Read the model definition and answer for the solid it produces. Units are mm, in the model's axes. A direction names the side the tool comes from. Give positions to 0.01 mm unless a question says otherwise; leave off trailing zeros. Loops run counter-clockwise (first coordinate to the right, second up) from the corner with the lowest first, then second, coordinate; pieces in that order, holes last.
(1) Straight lines are drawn through the part: probe 1 along Y at (x, z) = (-13, 12.75); probe 2 along X at (y, z) = (-15, 6); probe 3 along X at (y, z) = (-33.45, 27.5). For each, find the intervals that lie inside material, in ascending order.
(2) Which of the six approach directions +Z, -Z, +X, -X, +Y, -Y give full straight-line access (tool end or side, diameter ignored) to faces 1 (the face through (-14, -33.279, 27)), 2 (the face through (-4.076, -41.895, 27.395)), 3 (the face through (-6.434, 5.9, 3.914))?
(3) Determine the mould class of faces 4 (the face through (0, 25, 10)), 5 (the face through (-1.82, -23.22, 13.41)), 6 (the face through (8, -34.261, 25.7)), 7 (the face through (-15.674, -15.132, 9.86)) for opening direction Y: pulls with the +Y half, pulls with the -Y half, needs draft (parallel to the pull), parting line crosses it, or undercut.
(4) Each of these flat-tipped pins is pushed along its axis until it touches: P1, Ø14, axis at x = -0.5, y = 1.5, coming from the -Z side; P2, Ø6.5, axis at x = 8.5, z = 24.5, coming from the +Y side; P3, Ø3, axis at x = -2, y = -23, coming from the +Z side; P4, Ø13, axis at x = -6, y = 1, coming from the +Z side. Where does it stop, or does it pass through?
(5) Find section C-C, the plane x = -1. Write down the section's boundary in (y, z).
(6) Find section A-A, the plane z = 27.5. State how many separate pieces and enclosed holes the cut face has, then the cut area to 3 significant figures.
(7) Find section B-B, the plane y = -17. Write down the section's boundary in (x, z), then the cut area to 3 significant figures.
(8) Find section D-D, the plane z = 18.5. Write down the section's boundary in (x, y), then the cut area to 3 significant figures.
```python
from build123d import *

# Parameters (mm, degrees)
SKETCH1_W           = 42.62295082
SKETCH1_H           = 50
SKETCH1_R           = 2.677018134
BOSS_EXTRUDE1_DEPTH = 20
SKETCH2_R           = 8.73
CUT_EXTRUDE2_DEPTH  = 7.94
SKETCH3_R           = 2.2
CUT_EXTRUDE3_DEPTH  = 10
CUT_EXTRUDE4_START  = -7
CUT_EXTRUDE4_DEPTH  = 32.460095998
SKETCH7_W           = 42.62295082
SKETCH7_H           = 20
BOSS_EXTRUDE2_DEPTH = 18
SKETCH6_R           = 6.4
CUT_EXTRUDE5_DEPTH  = 52.992105017
BOSS_EXTRUDE5_DEPTH = 15
SKETCH10_R          = 1.55
CUT_EXTRUDE8_DEPTH  = 80.392562524


with BuildPart() as part:
    # Sketch1 → Boss-Extrude1 (new body)
    with BuildSketch(Plane.XY):
        Rectangle(SKETCH1_W, SKETCH1_H)
        with Locations((-13, -15.25)):
            Circle(SKETCH1_R, mode=Mode.SUBTRACT)
        with Locations(Location((13, -15.25, 0), (0, 0, 180))):
            Circle(SKETCH1_R, mode=Mode.SUBTRACT)
        with Locations((13, 15.25)):
            Circle(SKETCH1_R, mode=Mode.SUBTRACT)
        with Locations(Location((-13, 15.25, 0), (0, 0, 180))):
            Circle(SKETCH1_R, mode=Mode.SUBTRACT)
    extrude(amount=BOSS_EXTRUDE1_DEPTH)

    # Sketch2 → Cut-Extrude2 (cut)
    with BuildSketch(Plane.XY):
        Circle(SKETCH2_R)
    extrude(amount=CUT_EXTRUDE2_DEPTH, mode=Mode.SUBTRACT)

    # Sketch3 → Cut-Extrude3 (cut)
    with BuildSketch(Plane(origin=(0, 0, 0), x_dir=(-1, 0, 0), z_dir=(0, 0, -1))):
        with Locations((0, -20)):
            Circle(SKETCH3_R)
    extrude(amount=-CUT_EXTRUDE3_DEPTH, mode=Mode.SUBTRACT)

    # Sketch5 → Cut-Extrude4 (cut, through all)
    with BuildSketch(Plane(origin=(0, 0, 0), x_dir=(-1, 0, 0), z_dir=(0, 0, -1)).offset(CUT_EXTRUDE4_START)):
        Polygon((0, -15.727608008), (-3.7, -17.863804004), (-3.7, -22.136195996), (0, -24.272391992), (3.7, -22.136195996), (3.7, -17.863804004), align=None)
    extrude(amount=-CUT_EXTRUDE4_DEPTH, mode=Mode.SUBTRACT)

    # Sketch7 → Boss-Extrude2 (add)
    with BuildSketch(Plane.XZ.offset(25)):
        with Locations((0, 10)):
            Rectangle(SKETCH7_W, SKETCH7_H)
    extrude(amount=BOSS_EXTRUDE2_DEPTH)

    # Sketch6 → Cut-Extrude5 (cut, through all)
    with BuildSketch(Plane(origin=(0, 0, 0), x_dir=(-1, 0, 0), z_dir=(0, 0, -1))):
        with Locations((3.896856088, -32.824049036)):
            Circle(SKETCH6_R)
    extrude(amount=-CUT_EXTRUDE5_DEPTH, mode=Mode.SUBTRACT)

    # Sketch8 → Boss-Extrude5 (add)
    with BuildSketch(Plane.XY.offset(20)):
        with BuildLine():
            ThreePointArc((-10.280677785, -32.369273769), (-3.896856088, -26.424049036), (2.486965609, -32.369273769))
            Line((2.486965609, -32.369273769), (11.091790538, -32.369273769))
            Line((11.091790538, -32.369273769), (11.091790538, -31.387593744))
            Line((11.091790538, -31.387593744), (5.061469986, -31.387593744))
            ThreePointArc((5.061469986, -31.387593744), (-3.896856088, -23.751287061), (-12.855182162, -31.387593744))
            Line((-12.855182162, -31.387593744), (-18.885502714, -31.387593744))
            Line((-18.885502714, -31.387593744), (-18.885502714, -32.369273769))
            Line((-18.885502714, -32.369273769), (-10.280677785, -32.369273769))
        make_face()
        with BuildLine():
            Line((-10.280677785, -33.278824303), (-18.885502714, -33.278824303))
            Line((-18.885502714, -33.278824303), (-18.885502714, -34.260504328))
            Line((-18.885502714, -34.260504328), (-12.855182162, -34.260504328))
            ThreePointArc((-12.855182162, -34.260504328), (-3.896856088, -41.896811011), (5.061469986, -34.260504328))
            Line((5.061469986, -34.260504328), (11.091790538, -34.260504328))
            Line((11.091790538, -34.260504328), (11.091790538, -33.278824303))
            Line((11.091790538, -33.278824303), (2.486965609, -33.278824303))
            ThreePointArc((2.486965609, -33.278824303), (-3.896856088, -39.224049036), (-10.280677785, -33.278824303))
        make_face()
    extrude(amount=BOSS_EXTRUDE5_DEPTH)

    # Sketch10 → Cut-Extrude8 (cut, through all)
    with BuildSketch(Plane.XZ.offset(43)):
        with Locations(Location((-15.870502714, 27.5, 0), (0, 0, 90))):
            Circle(SKETCH10_R)
        with Locations(Location((8.071790538, 27.5, 0), (0, 0, 270))):
            Circle(SKETCH10_R)
    extrude(amount=-CUT_EXTRUDE8_DEPTH, mode=Mode.SUBTRACT)


solid = part.part
```
Entries:
1. probe 1: y = -43 to -17.93, -12.57 to 12.57, 17.93 to 25
1. probe 2: x = -21.31 to -15.67, -10.33 to 10.33, 15.67 to 21.31
1. probe 3: x = -18.89 to -17.42, -14.32 to -10.27, 2.47 to 6.52, 9.62 to 11.09
2. face 1: +Z, +X, -X
2. face 2: +Z, -Y
2. face 3: -Z
3. face 4: pulls with the +Y half
3. face 5: undercut
3. face 6: pulls with the -Y half
3. face 7: undercut
4. P1: stops at z = 7.94
4. P2: stops at y = -31.39
4. P3: stops at z = 35
4. P4: stops at z = 20
5. outline: (-43, 0) - (-38.53, 0) - (-38.53, 35) - (-41.42, 35) - (-41.42, 20) - (-43, 20) - close; (-27.12, 0) - (-21.96, 0) - (-21.96, 7) - (-23.7, 7) - (-23.7, 20) - (-24.23, 20) - (-24.23, 35) - (-27.12, 35) - close; (-18.04, 0) - (-8.67, 0) - (-8.67, 7.94) - (8.67, 7.94) - (8.67, 0) - (25, 0) - (25, 20) - (-16.3, 20) - (-16.3, 7) - (-18.04, 7) - close
6. separate pieces: 6
6. enclosed holes: 0
6. area: 136 mm2
7. outline: (-21.31, 0) - (-15.03, 0) - (-15.03, 20) - (-21.31, 20) - close; (-10.97, 0) - (10.97, 0) - (10.97, 20) - (2.2, 20) - (2.2, 7) - (-2.2, 7) - (-2.2, 20) - (-10.97, 20) - close; (15.03, 0) - (21.31, 0) - (21.31, 20) - (15.03, 20) - close
7. area: 633 mm2
8. outline: (-21.31, -43) - (21.31, -43) - (21.31, 25) - (-21.31, 25) - close; hole circle Ø5.35 at (-13, -15.25); hole circle Ø5.35 at (-13, 15.25); hole circle Ø12.8 at (-3.9, -32.82); hole (-3.7, -22.14) - (0, -24.27) - (3.7, -22.14) - (3.7, -17.86) - (0, -15.73) - (-3.7, -17.86) - close; hole circle Ø5.35 at (13, -15.25); hole circle Ø5.35 at (13, 15.25)
8. area: 2,630 mm2
